Geometry check sheet. Reference: drawing and pictorial views, mm from the part's lowest x, y, z. A direction names the side the tool comes from. Round coordinates to 2 decimals unless told otherwise and drop trailing zeros. Order: outer loops, then holes, each group sorted by start corner. A loop starts at its lowest first (then second) coordinate and runs counter-clockwise, first axis right, second up. Notation, with made-up numbers: (39.25, -6.75) -> (89.25, -6.75) arc R7 ccw to (89.25, -0.75) -> close; hole circle Ø4 at (-20.5, 34.5). An arc over 180 degrees is marked (long way). Put each result on its own line as item: value.
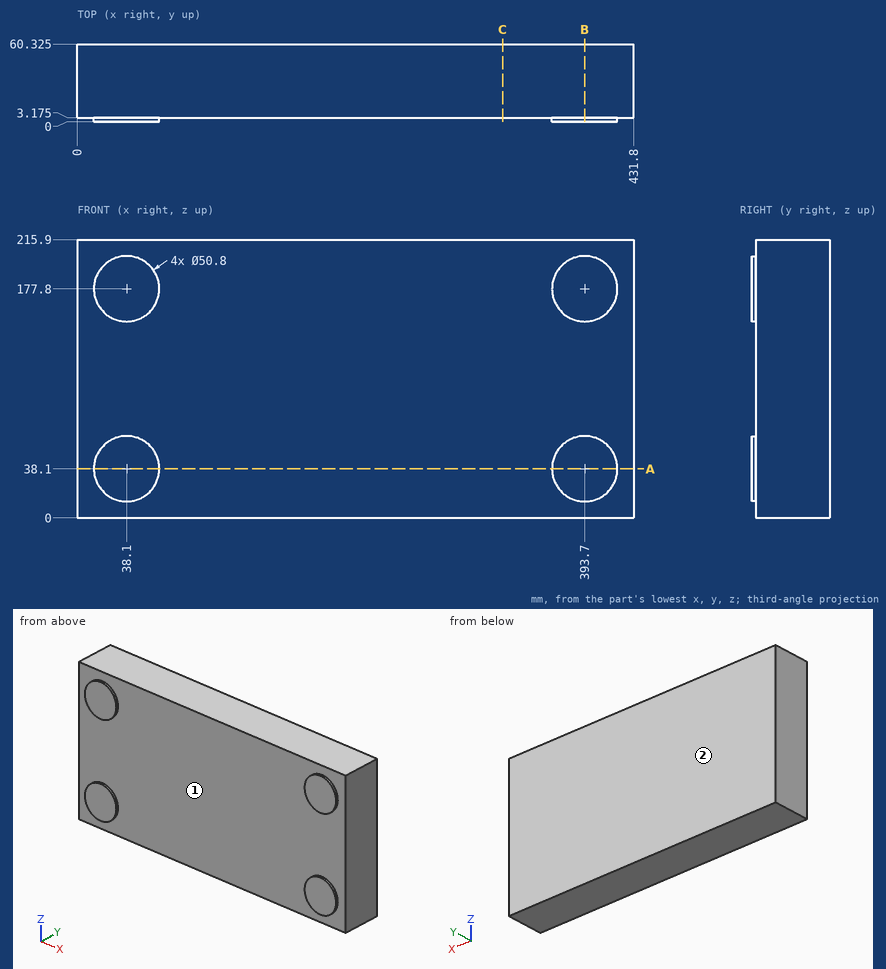
Item 1: Tool access check on the marked faces 1 and 2. Record the directions out of +Z, -Z, +X, -X, +Y, -Y that give a thin tool (end or side, any length) a straight path to the whole face; none if there is none.
Geometry check:
face 1: -Y
face 2: +Z, -Z, +X, -X, +Y
Item 2: Sectioned sample at B-B, the plane x = 393.7. Record the boundary of the cut face in (y, z) (3 decimals).
Geometry check:
outline: (0, 12.7) -> (3.175, 12.7) -> (3.175, 0) -> (60.325, 0) -> (60.325, 215.9) -> (3.175, 215.9) -> (3.175, 203.2) -> (0, 203.2) -> (0, 152.4) -> (3.175, 152.4) -> (3.175, 63.5) -> (0, 63.5) -> close
Item 3: Material ranges on line 1 along Y through (x, z) = (340, 88) (3 decimals), recorded low to high.
Geometry check:
line 1: 3.175 to 60.325
Item 4: Sectioned sample at C-C, the plane x = 330. Record the boundary of the cut face in (y, z) (3 decimals).
Geometry check:
outline: (3.175, 0) -> (60.325, 0) -> (60.325, 215.9) -> (3.175, 215.9) -> close
Item 5: Sectioned sample at A-A, the plane z = 38.1. Record the boundary of the cut face in (x, y) (3 decimals).
Geometry check:
outline: (0, 3.175) -> (12.7, 3.175) -> (12.7, 0) -> (63.5, 0) -> (63.5, 3.175) -> (368.3, 3.175) -> (368.3, 0) -> (419.1, 0) -> (419.1, 3.175) -> (431.8, 3.175) -> (431.8, 60.325) -> (0, 60.325) -> close
Item 6: Depth check by flat-ended pin: pin 1 Ø1 at (x, z) = (188.5, 163.5) entering from -Y (3 decimals). Enter the tip coordinate at first touch or a pass-through.
Geometry check:
pin 1: y = 3.175
